from build123d import *

# Parameters (mm, degrees)
SKETCH_1_R          = 2
EXTRUDE_1_DEPTH     = 2.5
FILLET_1_R          = 5
SKETCH_2_W          = 5
SKETCH_2_H          = 12
EXTRUDE_2_DEPTH     = 10
SKETCH_3_R          = 2
CUT_EXTRUDE_1_DEPTH = 48.172555581


with BuildPart() as part:
    # 草图1 → 凸台-拉伸1 (new, symmetric)
    with BuildSketch(Plane.XY):
        with BuildLine():
            Line((-25, -25), (25, -25))
            Line((25, -25), (25, -12))
            Line((25, -12), (20, -12))
            ThreePointArc((20, -12), (8, 0), (20, 12))
            Line((20, 12), (25, 12))
            Line((25, 12), (25, 25))
            Line((25, 25), (-25, 25))
            Line((-25, 25), (-25, 12))
            Line((-25, 12), (-20, 12))
            ThreePointArc((-20, 12), (-8, 0), (-20, -12))
            Line((-20, -12), (-25, -12))
            Line((-25, -12), (-25, -25))
        make_face()
        with Locations((-20, 20)):
            Circle(SKETCH_1_R, mode=Mode.SUBTRACT)
        with Locations((-20, -20)):
            Circle(SKETCH_1_R, mode=Mode.SUBTRACT)
        with Locations((20, 20)):
            Circle(SKETCH_1_R, mode=Mode.SUBTRACT)
        with Locations((20, -20)):
            Circle(SKETCH_1_R, mode=Mode.SUBTRACT)
    extrude(amount=EXTRUDE_1_DEPTH, both=True)

    # 圆角1
    fillet_1_edges = [part.edges().sort_by_distance(p)[0] for p in [
        (-25, 25, 0),
        (25, 25, 0),
        (25, -25, 0),
        (-25, -25, 0),
    ]]
    fillet(fillet_1_edges, radius=FILLET_1_R)

    # 草图2 → 凸台-拉伸2 (add)
    with BuildSketch(Plane.XY.offset(2.5)):
        with Locations((-10.5, 19)):
            Rectangle(SKETCH_2_W, SKETCH_2_H)
        with Locations((-0.5, -19)):
            Rectangle(SKETCH_2_W, SKETCH_2_H)
        with Locations((-0.5, 19)):
            Rectangle(SKETCH_2_W, SKETCH_2_H)
        with Locations((-10.5, -19)):
            Rectangle(SKETCH_2_W, SKETCH_2_H)
    extrude(amount=EXTRUDE_2_DEPTH)

    # 草图3 → 切除-拉伸1 (cut, through all)
    with BuildSketch(Plane.ZY.offset(13)):
        with Locations(Location((8.5, 19, 0), (0, 0, 270))):
            Circle(SKETCH_3_R)
        with Locations(Location((8.5, -19, 0), (0, 0, 270))):
            Circle(SKETCH_3_R)
    extrude(amount=-CUT_EXTRUDE_1_DEPTH, mode=Mode.SUBTRACT)


solid = part.part
Could you check a few things on this model? Use its own coordinates, in mm. A direction names the side the tool comes from. Give positions to 0.01 mm unless a question says otherwise; leave off trailing zeros. Order: outer loops, then holes, each group sorted by start corner. A loop starts at its lowest first (then second) coordinate and runs counter-clockwise, first axis right, second up.
1. Which directions (+Z, -Z, +X, -X, +Y, -Y) give clear straight access to the entire face, cutting with the end or side of a thin tool? Please do faces 4 (the flat face through (-13, -19, 6)), 5 (the flat face through (22, 12, 0)), 6 (the flat face through (-11, 13, 7)).
Answers below:
face 4: +Z, -X, +Y, -Y
face 5: +Z, -Z, +X
face 6: +Z, +X, -X
2. For pin 1 (5 mm diameter, centred on y = -18, z = 5.5, fed in from +X); pin 2 (4 mm diameter, centred on x = -23, z = 0, fed in from +Y); pin 3 (5 mm diameter, centred on y = -18, z = 5.5, fed in from -X), each with a flat end and sliding along its axis, tell me the tip position at first contact or that it passes through.
Answers below:
pin 1: stops at x = 2
pin 2: stops at y = 24.9
pin 3: stops at x = -13
3. Suppose I cut it at D-D (x = -21). Write out the boundary of the cut face in (y, z), plus the area to 3 significant figures.
Answers below:
outline: (-24.9, -2.5) - (-21.73, -2.5) - (-21.73, 2.5) - (-24.9, 2.5) - close; (-18.27, -2.5) - (-12, -2.5) - (-12, 2.5) - (-18.27, 2.5) - close; (12, -2.5) - (18.27, -2.5) - (18.27, 2.5) - (12, 2.5) - close; (21.73, -2.5) - (24.9, -2.5) - (24.9, 2.5) - (21.73, 2.5) - close
area: 94.3 mm2
4. Thinking about a two-plate mould opening in Z: for faces 1 (the cylindrical face through (-0.535, -17.526, 9.852)), 2 (the flat face through (0, 0, -2.5)), 3 (the cylindrical face through (-8, 0, 0)), which applies, +Z half, -Z half, draft (parallel to the pull), parting line (faces both ways), or undercut?
Answers below:
face 1: undercut
face 2: -Z half
face 3: draft
5. I need wall thicknesses on L1, parallel to Y at x = -20, z = 1.2; L2, parallel to X at y = 16, z = 10; L3, parallel to Y at x = -11, z = 4.5. Which ranges of each line are inside material? Lowest first, please.
Answers below:
L1: y = -25 to -22, -18 to -12, 12 to 18, 22 to 25
L2: x = -13 to -8, -3 to 2
L3: y = -25 to -13, 13 to 25
6. Suppose I cut it at A-A (x = -10). Write out the boundary of the cut face in (y, z).
Answers below:
outline: (-25, -2.5) - (-6.63, -2.5) - (-6.63, 2.5) - (-13, 2.5) - (-13, 12.5) - (-25, 12.5) - close; (6.63, -2.5) - (25, -2.5) - (25, 12.5) - (13, 12.5) - (13, 2.5) - (6.63, 2.5) - close; hole circle Ø4 at (-19, 8.5); hole circle Ø4 at (19, 8.5)
7. Suppose I cut it at B-B (z = 8.5). State how many separate pieces and enclosed holes the cut face has, plus the area to 3 significant figures.
Answers below:
separate pieces: 8
enclosed holes: 0
area: 160 mm2
8. Suppose I cut it at C-C (y = -19). Write out the boundary of the cut face in (x, z).
Answers below:
outline: (-25, -2.5) - (-21.73, -2.5) - (-21.73, 2.5) - (-25, 2.5) - close; (-18.27, -2.5) - (18.27, -2.5) - (18.27, 2.5) - (2, 2.5) - (2, 6.5) - (-3, 6.5) - (-3, 2.5) - (-8, 2.5) - (-8, 6.5) - (-13, 6.5) - (-13, 2.5) - (-18.27, 2.5) - close; (-13, 10.5) - (-8, 10.5) - (-8, 12.5) - (-13, 12.5) - close; (-3, 10.5) - (2, 10.5) - (2, 12.5) - (-3, 12.5) - close; (21.73, -2.5) - (25, -2.5) - (25, 2.5) - (21.73, 2.5) - close
